```python
from build123d import *

# Parameters (mm, degrees)
F1_DEPTH = 101.6
F3_DEPTH = 1.0162968718


# Not quite as in the source:
# - ends of sketch curves that miss each other by under 0.0002 mm in the source are joined


with BuildPart() as f1:
    # F0 (on Right) → F1 (new body, symmetric)
    with BuildSketch(Plane.YZ):
        with BuildLine():
            Line((-13.9794936462, -2.032), (-13.9794936462, -5.5877193844))
            ThreePointArc((-13.9794936462, -5.5877193844), (-13.384185281, -7.0242872241), (-11.9474936901, -7.6192968718))
            Line((-11.9474936901, -7.6192968718), (11.9474936901, -7.6192968718))
            ThreePointArc((11.9474936901, -7.6192968718), (13.3841865534, -7.024285952), (13.9794936469, -5.5877157858))
            Line((13.9794936469, -5.5877157858), (13.9794936469, -2.0319964014))
            ThreePointArc((13.9794936469, -2.0319964014), (14.2772790988, -1.313078725), (14.9961967752, -1.0152932732))
            Line((14.9961967752, -1.0152932732), (17.7780878922, -1.0152932732))
            Line((17.7780878922, -1.0152932732), (17.7780878922, 0))
            Line((17.7780878922, 0), (14.9923725588, 0))
            ThreePointArc((14.9923725588, 0), (13.5581523434, -0.5963598833), (12.9641968184, -2.0315774874))
            Line((12.9641968184, -2.0315774874), (12.9641968184, -5.5872968718))
            ThreePointArc((12.9641968184, -5.5872968718), (12.6664113666, -6.3062145482), (11.9474936901, -6.604))
            Line((11.9474936901, -6.604), (-11.9474936901, -6.604))
            ThreePointArc((-11.9474936901, -6.604), (-12.6664113666, -6.3062145482), (-12.9641968184, -5.5872968718))
            Line((-12.9641968184, -5.5872968718), (-12.9641968184, -2.0315774874))
            ThreePointArc((-12.9641968184, -2.0315774874), (-13.5595051836, -0.5950096476), (-14.9961967744, 0))
            Line((-14.9961967744, 0), (-17.7819121078, 0))
            Line((-17.7819121078, 0), (-17.7819121078, -1.0152932732))
            Line((-17.7819121078, -1.0152932732), (-14.9961967744, -1.0152932732))
            ThreePointArc((-14.9961967744, -1.0152932732), (-14.277279098, -1.3130823236), (-13.9794936462, -2.032))
        make_face()
    extrude(amount=F1_DEPTH, both=True)

    # F2 (on face) → F3 (cut, through all)
    with BuildSketch(Plane.XY.offset(-6.604)):
        with BuildLine():
            Line((-5.715, -3.175), (5.715, -3.175))
            ThreePointArc((5.715, -3.175), (8.89, 0), (5.715, 3.175))
            Line((5.715, 3.175), (-5.715, 3.175))
            ThreePointArc((-5.715, 3.175), (-8.89, 0), (-5.715, -3.175))
        make_face()
        with BuildLine():
            Line((19.685, -3.175), (31.115, -3.175))
            ThreePointArc((31.115, -3.175), (34.29, 0), (31.115, 3.175))
            Line((31.115, 3.175), (19.685, 3.175))
            ThreePointArc((19.685, 3.175), (16.51, 0), (19.685, -3.175))
        make_face()
        with BuildLine():
            Line((45.085, -3.175), (56.515, -3.175))
            ThreePointArc((56.515, -3.175), (59.69, 0), (56.515, 3.175))
            Line((56.515, 3.175), (45.085, 3.175))
            ThreePointArc((45.085, 3.175), (41.91, 0), (45.085, -3.175))
        make_face()
        with BuildLine():
            Line((70.485, -3.175), (81.915, -3.175))
            ThreePointArc((81.915, -3.175), (85.09, 0), (81.915, 3.175))
            Line((81.915, 3.175), (70.485, 3.175))
            ThreePointArc((70.485, 3.175), (67.31, 0), (70.485, -3.175))
        make_face()
        with BuildLine():
            Line((95.885, -3.175), (107.315, -3.175))
            ThreePointArc((107.315, -3.175), (110.49, 0), (107.315, 3.175))
            Line((107.315, 3.175), (95.885, 3.175))
            ThreePointArc((95.885, 3.175), (92.71, 0), (95.885, -3.175))
        make_face()
        with BuildLine():
            Line((-19.685, 3.175), (-31.115, 3.175))
            ThreePointArc((-31.115, 3.175), (-34.29, 0), (-31.115, -3.175))
            Line((-31.115, -3.175), (-19.685, -3.175))
            ThreePointArc((-19.685, -3.175), (-16.51, 0), (-19.685, 3.175))
        make_face()
        with BuildLine():
            Line((-45.085, 3.175), (-56.515, 3.175))
            ThreePointArc((-56.515, 3.175), (-59.69, 0), (-56.515, -3.175))
            Line((-56.515, -3.175), (-45.085, -3.175))
            ThreePointArc((-45.085, -3.175), (-41.91, 0), (-45.085, 3.175))
        make_face()
        with BuildLine():
            Line((-70.485, 3.175), (-81.915, 3.175))
            ThreePointArc((-81.915, 3.175), (-85.09, 0), (-81.915, -3.175))
            Line((-81.915, -3.175), (-70.485, -3.175))
            ThreePointArc((-70.485, -3.175), (-67.31, 0), (-70.485, 3.175))
        make_face()
        with BuildLine():
            Line((-95.885, 3.175), (-107.315, 3.175))
            ThreePointArc((-107.315, 3.175), (-110.49, 0), (-107.315, -3.175))
            Line((-107.315, -3.175), (-95.885, -3.175))
            ThreePointArc((-95.885, -3.175), (-92.71, 0), (-95.885, 3.175))
        make_face()
    extrude(amount=-F3_DEPTH, mode=Mode.SUBTRACT)


solid = f1.part
```
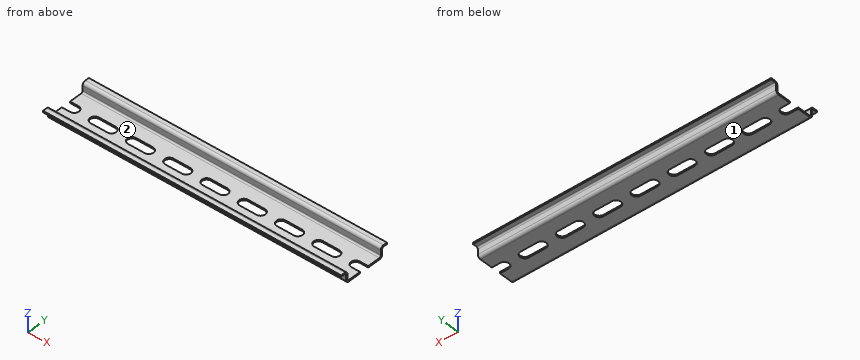
Here's how the part is built. I have some questions about the finished solid (model axes, mm). Face numbers are marked on the shaded views. A direction names the side the tool comes from. Coordinates: 2 decimals unless noted, no trailing zeros. Order: outer loops, then holes, each group sorted by start corner. A loop starts at its lowest first (then second) coordinate and runs counter-clockwise, first axis right, second up. Notation, with made-up numbers: (29.5, -28.5) - (70.5, -28.5) arc R23 cw to (70.5, 4.5) - close; hole circle Ø1 at (57.5, 76.25). An arc over 180 degrees is marked (long way). One line per question, with ' | ' between items. Start each with the question number.
1. If we section it at A-A (y = 0): Give the number of separate pieces and of enclosed holes in the cut face, and give its area (3 significant figures).
2. I'm going to push flat-ended pins straight in: pin 1 Ø0.8 at (x, z) = (98, -7) entering from +Y; pin 2 Ø0.8 at (x, y) = (4, 16) entering from -Z; pin 3 Ø0.8 at (x, z) = (-53, -7.5) entering from +Y. Where does each tip first touch, or does it pass through?
3. Please list where these lines run through material, in increasing order: line 1 along Y through (x, z) = (-5.5, -3.5); line 2 along Z through (x, y) = (51, -10.5); line 3 along Y through (x, z) = (68, -6). Write a range as [from, to].
4. If we section it at C-C (z = -3.75): Write out the boundary of the cut face in (x, y), and give its area (3 significant figures).
5. If we section it at B-B (x = 28.5): Write out the boundary of the cut face in (y, z) (1 decimal).
6. Which directions (+Z, -Z, +X, -X, +Y, -Y) give clear straight access to the entire face, cutting with the end or side of a thin tool? Please do the marked faces 1 and 2.
Model answer:
1) separate pieces: 8 | enclosed holes: 0 | area: 61.9 mm²
2) pin 1: stops at y = 13.71 | pin 2: stops at z = -1.02 | pin 3: stops at y = 13.3
3) line 1: y = [-13.98, -12.96], [12.96, 13.98] | line 2: z = [-7.62, -6.6] | line 3: y = [-13.94, -12.88], [12.88, 13.94]
4) outline: (-101.6, -13.98) - (101.6, -13.98) - (101.6, -12.96) - (-101.6, -12.96) - close; (-101.6, 12.96) - (101.6, 12.96) - (101.6, 13.98) - (-101.6, 13.98) - close | area: 413 mm²
5) outline: (-17.8, -1) - (-15, -1) arc R1 cw to (-14, -2) - (-14, -5.6) arc R2 ccw to (-11.9, -7.6) - (-3.2, -7.6) - (-3.2, -6.6) - (-11.9, -6.6) arc R1 cw to (-13, -5.6) - (-13, -2) arc R2 ccw to (-15, 0) - (-17.8, 0) - close; (3.2, -7.6) - (11.9, -7.6) arc R2 ccw to (14, -5.6) - (14, -2) arc R1 cw to (15, -1) - (17.8, -1) - (17.8, 0) - (15, 0) arc R2 ccw to (13, -2) - (13, -5.6) arc R1 cw to (11.9, -6.6) - (3.2, -6.6) - close
6) face 1: -Z, +X, -X, +Y, -Y | face 2: +Z, +X, -X
